Work out the finished part from the listing and answer in its coordinate system (mm). A direction names the side the tool comes from. Round coordinates to 2 decimals unless told otherwise and drop trailing zeros. Loops run counter-clockwise (first coordinate to the right, second up) from the corner with the lowest first, then second, coordinate; pieces in that order, holes last. Notation, with made-up numbers: M -26.75,3 L -16.75,3 A21 cw -16.75,31 Z; hole C -15.5,53.25 d11. An arc over 180 degrees is marked long. One line per item, written item: value.
```python
from build123d import *

# Parameters (mm, degrees)
SKETCH_1_W        = 15
SKETCH_1_H        = 40
EXTRUDE_2_DEPTH   = 30
SKETCH_1_H_2      = 10
EXTRUDE_2_2_DEPTH = 30
EXTRUDE_2_3_DEPTH = 30
SKETCH_1_6_W      = 15
SKETCH_1_6_H      = 20
EXTRUDE_4_DEPTH   = 15
SKETCH_1_7_R      = 5
EXTRUDE_5_DEPTH   = 10


with BuildPart() as part:
    # Sketch 1 → Extrude 2 (new body)
    with BuildSketch(Plane(origin=(0, 0, 0), x_dir=(1, 0, 0), z_dir=(0, 1, 0))):
        with Locations((-43.568318821, -33.556262559)):
            Rectangle(SKETCH_1_W, SKETCH_1_H)
    extrude(amount=EXTRUDE_2_DEPTH)



with BuildPart() as body_2:
    # Sketch 1 → Extrude 2 2 (new body)
    with BuildSketch(Plane(origin=(0, 0, 0), x_dir=(1, 0, 0), z_dir=(0, 1, 0))):
        with Locations((21.431681179, -48.556262559)):
            Rectangle(SKETCH_1_W, SKETCH_1_H_2)
    extrude(amount=EXTRUDE_2_2_DEPTH)



with BuildPart() as body_3:
    # Sketch 1 → Extrude 2 3 (new body)
    with BuildSketch(Plane(origin=(0, 0, 0), x_dir=(1, 0, 0), z_dir=(0, 1, 0))):
        with Locations((21.431681179, -18.556262559)):
            Rectangle(SKETCH_1_W, SKETCH_1_H_2)
    extrude(amount=EXTRUDE_2_3_DEPTH)


with BuildPart() as body_2_1:
    add(body_2.part)

    add(body_3.part)  # Extrude 4 merges body 3
    # Sketch 1_6 → Extrude 4 (add)
    with BuildSketch(Plane(origin=(0, 0, 0), x_dir=(1, 0, 0), z_dir=(0, 1, 0))):
        with Locations((21.431681179, -33.556262559)):
            Rectangle(SKETCH_1_6_W, SKETCH_1_6_H)
    extrude(amount=EXTRUDE_4_DEPTH)


with BuildPart() as part_1:
    add(part.part)

    add(body_2_1.part)  # Extrude 5 merges body 2
    # Sketch 1_7 → Extrude 5 (add)
    with BuildSketch(Plane(origin=(0, 0, 0), x_dir=(1, 0, 0), z_dir=(0, 1, 0))):
        Polygon((13.931681179, -13.556262559), (-36.068318821, -13.556262559), (-36.068318821, -53.556262559), (13.931681179, -53.556262559), (13.931681179, -43.556262559), (13.931681179, -23.556262559), align=None)
        with Locations(Location((-21.068318821, -33.556262559, 0), (0, 0, 270))):
            Circle(SKETCH_1_7_R, mode=Mode.SUBTRACT)
        with Locations(Location((-1.068318821, -33.556262559, 0), (0, 0, 270))):
            Circle(SKETCH_1_7_R, mode=Mode.SUBTRACT)
    extrude(amount=EXTRUDE_5_DEPTH)


solid = part_1.part
```
1) Find section A-A (y = 27.75). Give the vertices of the cut face in (x, z).
Check values:
outline: M -51.07,13.56 L -36.07,13.56 L -36.07,53.56 L -51.07,53.56 Z; M 13.93,13.56 L 28.93,13.56 L 28.93,23.56 L 13.93,23.56 Z; M 13.93,43.56 L 28.93,43.56 L 28.93,53.56 L 13.93,53.56 Z
2) Each of these flat-tipped pins is pushed along its axis until it touches: pin 1 (3 mm diameter, centred on x = -34, y = 26, fed in from -Z); pin 2 (12 mm diameter, centred on x = 21.5, z = 34, fed in from +Y). Where does it stop, or does it pass through?
Check values:
pin 1: through
pin 2: y = 15
3) Find the intervals of material crossed by probe 1 along X at (y, z) = (5.75, 37); probe 2 along X at (y, z) = (2, 36); probe 3 along Z at (x, y) = (22, 27), in increasing order. Write a range as from..to.
Check values:
probe 1: -51.07..-24.69, -17.44..-4.69, 2.56..28.93
probe 2: -51.07..-25.43, -16.71..-5.43, 3.29..28.93
probe 3: 13.56..23.56, 43.56..53.56
4) For faces 4 (the face through (21, 22, 43.556)), 5 (the face through (-11, 10, 33)), 6 (the face through (-51.068, 15, 34)), determine the directions among +Z, -Z, +X, -X, +Y, -Y from which every point of the face is accessible in a straight line to the end or side of a thin tool.
Check values:
face 4: +X, +Y
face 5: +Z, -Z, +Y
face 6: +Z, -Z, -X, +Y, -Y
5) Find section B-B (y = 14). Give the vertices of the cut face in (x, z).
Check values:
outline: M -51.07,13.56 L -36.07,13.56 L -36.07,53.56 L -51.07,53.56 Z; M 13.93,13.56 L 28.93,13.56 L 28.93,53.56 L 13.93,53.56 Z
6) Find section C-C (z = 24.5). Give the vertices of the cut face in (x, y).
Check values:
outline: M -51.07,0 L 28.93,0 L 28.93,15 L 13.93,15 L 13.93,10 L -36.07,10 L -36.07,30 L -51.07,30 Z
7) The mould has two halves that part along Z. Classify faces 1 (the face through (-11, 8, 13.556)), 2 (the face through (-44, 30, 33)), 3 (the face through (-16.11, 4.93, 32.91)): +Z half, -Z half, draft (parallel to the pull), parting line (faces both ways), or undercut.
Check values:
face 1: -Z half
face 2: draft
face 3: undercut
8) Find section D-D (x = 22.5). Give the vertices of the cut face in (y, z), then the cut area to 3 significant figures.
Check values:
outline: M 0,13.56 L 30,13.56 L 30,23.56 L 15,23.56 L 15,43.56 L 30,43.56 L 30,53.56 L 0,53.56 Z
area: 900 mm2
